The model under review builds one solid part; all positions refer to its coordinate system, in mm. Give positions to 0.01 mm unless a question says otherwise; leave off trailing zeros. Write each loop counter-clockwise with the first axis right and the second up, starting at its lowest first coordinate (ties: lowest second). Pieces come first, ordered by that corner, then holes. Notation, with made-up numbers: (8, -17.5) - (66, -17.5) arc R30 cw to (66, 5.5) - close; hole circle Ø4 at (31, 21). An arc over 180 degrees is marked (long way). Write item = value, one per line.
```python
from build123d import *

# Parameters (mm, degrees)
F0_W     = 85
F0_H     = 74
F1_DEPTH = 25


with BuildPart() as f1:
    # F0 (on Front) → F1 (new body)
    with BuildSketch(Plane.XZ):
        with Locations((0, 37)):
            Rectangle(F0_W, F0_H)
        Polygon((40.5, 2), (-40.5, 2), (-40.5, 26.5), (-20.3, 26.5), (-20.3, 28.5), (-40.5, 28.5), (-40.5, 35), (-32.1, 35), (-32.1, 33.3), (-27.1, 33.3), (-27.1, 37), (-40.5, 37), (-40.5, 72), (38.9, 72), (38.9, 32.2), (40.5, 32.2), (40.5, 30.2), (38.9, 30.2), (38.9, 28), (34, 28), (34, 30.2), (8.9, 30.2), (8.9, 28), (4, 28), (4, 30.2), (2.4, 30.2), (2.4, 32.2), (4, 32.2), (4, 39.5), (-15.7, 39.5), (-15.7, 30.8), (-14.8, 30.8), (-14.8, 28.5), (-15.6, 28.5), (-15.6, 26.5), (40.5, 26.5), align=None, mode=Mode.SUBTRACT)
    extrude(amount=F1_DEPTH)


solid = f1.part
```
1. Insertion check: P1, Ø10, axis at x = -18.5, z = 48.5, coming from the -Y side. The pin has a flat end and moves straight along its axis. Give the tip position at first contact, or say it passes through.
Findings below:
P1 = through
2. Take a section at C-C on x = -18. Give the boundary of the cut face in (y, z), and give its area (3 significant figures).
Findings below:
outline = (-25, 0) - (0, 0) - (0, 2) - (-25, 2) - close; (-25, 72) - (0, 72) - (0, 74) - (-25, 74) - close
area = 100 mm²
3. Take a section at B-B on x = -0.5. Give the boundary of the cut face in (y, z).
Findings below:
outline = (-25, 0) - (0, 0) - (0, 2) - (-25, 2) - close; (-25, 26.5) - (0, 26.5) - (0, 39.5) - (-25, 39.5) - close; (-25, 72) - (0, 72) - (0, 74) - (-25, 74) - close
4. Take a section at A-A on z = 68. Give the boundary of the cut face in (x, y), and give its area (3 significant figures).
Findings below:
outline = (-42.5, -25) - (-40.5, -25) - (-40.5, 0) - (-42.5, 0) - close; (38.9, -25) - (42.5, -25) - (42.5, 0) - (38.9, 0) - close
area = 140 mm²
5. For line 1 (Z direction, x = -32.5, y = -11.5); line 2 (Z direction, x = 9, y = -1.75); line 3 (Z direction, x = 1.5, y = -8.5), list the stretches that pass through material, from the lowest coordinate up. Write a range as from..to.
Findings below:
line_1 = 0..2, 26.5..28.5, 35..37, 72..74
line_2 = 0..2, 26.5..30.2, 72..74
line_3 = 0..2, 26.5..39.5, 72..74
6. Draft analysis for pull direction Z (two halves, no side actions). For faces 1 (the flat face through (-1, -12, 74)), 2 (the flat face through (34, -12, 29)), state which applies: +Z half, -Z half, draft (parallel to the pull), parting line (faces both ways), or undercut.
Findings below:
face_1 = +Z half
face_2 = undercut
7. Take a section at D-D on x = 23. Give the boundary of the cut face in (y, z), and give its area (4 significant figures).
Findings below:
outline = (-25, 0) - (0, 0) - (0, 2) - (-25, 2) - close; (-25, 26.5) - (0, 26.5) - (0, 30.2) - (-25, 30.2) - close; (-25, 72) - (0, 72) - (0, 74) - (-25, 74) - close
area = 192.5 mm²
